from build123d import *

# Parameters (mm, degrees)
SKETCH1_W           = 241.3
SKETCH1_H           = 38.1
BOSS_EXTRUDE1_DEPTH = 2.54
SKETCH2_R           = 2.54
CUT_EXTRUDE1_DEPTH  = 2.54
LPATTERN1_COUNT     = 19
LPATTERN1_PITCH     = 12.7


with BuildPart() as part:
    # Sketch1 → Boss-Extrude1 (new body)
    with BuildSketch(Plane(origin=(0, 0, 0), x_dir=(1, 0, 0), z_dir=(0, 1, 0))):
        Rectangle(SKETCH1_W, SKETCH1_H)
    extrude(amount=BOSS_EXTRUDE1_DEPTH)

    # Sketch2 → Cut-Extrude1 (cut)
    with BuildSketch(Plane(origin=(0, 2.54, 0), x_dir=(1, 0, 0), z_dir=(0, 1, 0))):
        with Locations(Location((-114.3, 0, 0), (0, 0, 270))):
            Circle(SKETCH2_R)
    cut_extrude1 = extrude(amount=-CUT_EXTRUDE1_DEPTH, mode=Mode.SUBTRACT)

    # LPattern1: Cut-Extrude1 ×19
    with Locations(*[(i * LPATTERN1_PITCH, 0, 0) for i in range(1, LPATTERN1_COUNT)]):
        add(cut_extrude1, mode=Mode.SUBTRACT)


solid = part.part
Build history of the part. All positions in model axes, mm. Round coordinates to 2 decimals unless told otherwise and drop trailing zeros. Write each loop counter-clockwise with the first axis right and the second up, starting at its lowest first coordinate (ties: lowest second). Pieces come first, ordered by that corner, then holes. Notation, with made-up numbers: (60, 37.25) - (112, 37.25) arc R24 ccw to (112, 59.25) - close; hole circle Ø5 at (52.25, 5.25). An arc over 180 degrees is marked (long way). Use CSV: the item, a comma, the result in double quotes.
(1) Band-saw the part on A-A (x = -25.4). Write the cut outline in (y, z).
Response:
outline,"(0, -19.05) - (2.54, -19.05) - (2.54, -2.54) - (0, -2.54) - close; (0, 2.54) - (2.54, 2.54) - (2.54, 19.05) - (0, 19.05) - close"
(2) Band-saw the part on B-B (y = 0.85). Give the number of separate pieces and of enclosed holes in the cut face, plus the area to 3 significant figures.
Response:
separate pieces,"1"
enclosed holes,"19"
area,"8,810 mm²"
(3) Mould opens along Z. For faces 1 (the flat face through (-2, 2.54, -5)), 2 (the cylindrical face through (-48.28, 1.29, -0.33)) say: pulls with the +Z half, pulls with the -Z half, needs draft (parallel to the pull), parting line crosses it, or undercut.
Response:
face 1,"needs draft"
face 2,"undercut"
(4) Pin check, flat tip, straight feed: P1, Ø4, axis at x = 76.2, z = 0, coming from the +Y side. Stop position of the tip, or through.
Response:
P1,"through"
(5) Wall check: line 1 (Z direction, x = 102, y = 1.3); line 2 (Z direction, x = 14, y = 0.6). Give the ranges that are in metal, low to high.
Response:
line 1,"-19.05 to -2.51, 2.51 to 19.05"
line 2,"-19.05 to -2.18, 2.18 to 19.05"
